from build123d import *

# Parameters (mm, degrees)
EXTRUDE_1_DEPTH     = 1.2
SKETCH_2_R          = 1.375
CUT_EXTRUDE_1_DEPTH = 1.2
SKETCH_3_W          = 6
SKETCH_3_H          = 13
EXTRUDE_2_DEPTH     = 5
SKETCH_4_W          = 6
SKETCH_4_H          = 5
EXTRUDE_3_DEPTH     = 0.3
SKETCH_5_W          = 14.5
SKETCH_5_H          = 7
EXTRUDE_4_DEPTH     = 9
SKETCH_6_W          = 13
SKETCH_6_H          = 6
EXTRUDE_5_DEPTH     = 6
SKETCH_11_W         = 51.4
SKETCH_11_H         = 5.1
EXTRUDE_9_DEPTH     = 8.5
SKETCH_12_W         = 6.2
SKETCH_12_H         = 6.2
EXTRUDE_10_DEPTH    = 3.5
SKETCH_13_R         = 1.75
EXTRUDE_11_DEPTH    = 1.5
SKETCH_15_R         = 2.75
SKETCH_15_R_2       = 1.55
EXTRUDE_13_DEPTH    = 2
SKETCH_16_W         = 51.4
SKETCH_16_H         = 5.1
EXTRUDE_14_DEPTH    = 9


with BuildPart() as part:
    # 草图1 → 凸台-拉伸1 (new body)
    with BuildSketch(Plane(origin=(0, 0, 0), x_dir=(1, 0, 0), z_dir=(0, 1, 0))):
        with BuildLine():
            Line((-29.5, 15), (29.5, 15))
            ThreePointArc((29.5, 15), (31.621320344, 14.121320344), (32.5, 12))
            Line((32.5, 12), (32.5, -12))
            ThreePointArc((32.5, -12), (31.621320344, -14.121320344), (29.5, -15))
            Line((29.5, -15), (-29.5, -15))
            ThreePointArc((-29.5, -15), (-31.621320344, -14.121320344), (-32.5, -12))
            Line((-32.5, -12), (-32.5, 12))
            ThreePointArc((-32.5, 12), (-31.621320344, 14.121320344), (-29.5, 15))
        make_face()
    extrude(amount=EXTRUDE_1_DEPTH)

    # 草图2 → 切除-拉伸1 (cut)
    with BuildSketch(Plane(origin=(0, 1.2, 0), x_dir=(1, 0, 0), z_dir=(0, 1, 0))):
        with Locations(Location((29, -11.5, 0), (0, 0, 270))):
            Circle(SKETCH_2_R)
        with Locations(Location((29, 11.5, 0), (0, 0, 270))):
            Circle(SKETCH_2_R)
        with Locations(Location((-29, -11.5, 0), (0, 0, 270))):
            Circle(SKETCH_2_R)
        with Locations(Location((-29, 11.5, 0), (0, 0, 270))):
            Circle(SKETCH_2_R)
    extrude(amount=-CUT_EXTRUDE_1_DEPTH, mode=Mode.SUBTRACT)

    # 草图3 → 凸台-拉伸2 (add)
    with BuildSketch(Plane(origin=(0, 1.2, 0), x_dir=(1, 0, 0), z_dir=(0, 1, 0))):
        with Locations((21.5, -8.5)):
            Rectangle(SKETCH_3_W, SKETCH_3_H)
    extrude(amount=EXTRUDE_2_DEPTH)

    # 草图4 → 凸台-拉伸3 (add)
    with BuildSketch(Plane.XY.offset(15)):
        with Locations((21.5, 3.7)):
            Rectangle(SKETCH_4_W, SKETCH_4_H)
    extrude(amount=EXTRUDE_3_DEPTH)

    # 草图5 → 凸台-拉伸4 (add)
    with BuildSketch(Plane(origin=(0, 1.2, 0), x_dir=(1, 0, 0), z_dir=(0, 1, 0))):
        with Locations((-0.75, -11.5)):
            Rectangle(SKETCH_5_W, SKETCH_5_H)
    extrude(amount=EXTRUDE_4_DEPTH)

    # 草图6 → 凸台-拉伸5 (add)
    with BuildSketch(Plane(origin=(0, 1.2, 0), x_dir=(1, 0, 0), z_dir=(0, 1, 0))):
        with Locations((-17, -12)):
            Rectangle(SKETCH_6_W, SKETCH_6_H)
    extrude(amount=EXTRUDE_5_DEPTH)

    # 草图11 → 凸台-拉伸9 (add)
    with BuildSketch(Plane.XZ):
        with Locations((-0.05, -11.55)):
            Rectangle(SKETCH_11_W, SKETCH_11_H)
    extrude(amount=EXTRUDE_9_DEPTH)

    # 草图12 → 凸台-拉伸10 (add)
    with BuildSketch(Plane(origin=(0, 1.2, 0), x_dir=(1, 0, 0), z_dir=(0, 1, 0))):
        with Locations((-15.4, 1.4)):
            Rectangle(SKETCH_12_W, SKETCH_12_H)
    extrude(amount=EXTRUDE_10_DEPTH)

    # 草图13 → 凸台-拉伸11 (add)
    with BuildSketch(Plane(origin=(0, 4.7, 0), x_dir=(1, 0, 0), z_dir=(0, 1, 0))):
        with Locations(Location((-15.4, 1.4, 0), (0, 0, 270))):
            Circle(SKETCH_13_R)
    extrude(amount=EXTRUDE_11_DEPTH)

    # 草图15 → 凸台-拉伸13 (add)
    with BuildSketch(Plane.XY.offset(15.3)):
        with Locations(Location((21.5, 3.7, 0), (0, 0, 114.619977329))):
            Circle(SKETCH_15_R)
        with Locations((21.5, 3.7)):
            Circle(SKETCH_15_R_2, mode=Mode.SUBTRACT)
    extrude(amount=EXTRUDE_13_DEPTH)

    # 草图16 → 凸台-拉伸14 (add)
    with BuildSketch(Plane(origin=(0, 1.2, 0), x_dir=(1, 0, 0), z_dir=(0, 1, 0))):
        with Locations((-0.05, 11.55)):
            Rectangle(SKETCH_16_W, SKETCH_16_H)
    extrude(amount=EXTRUDE_14_DEPTH)


solid = part.part
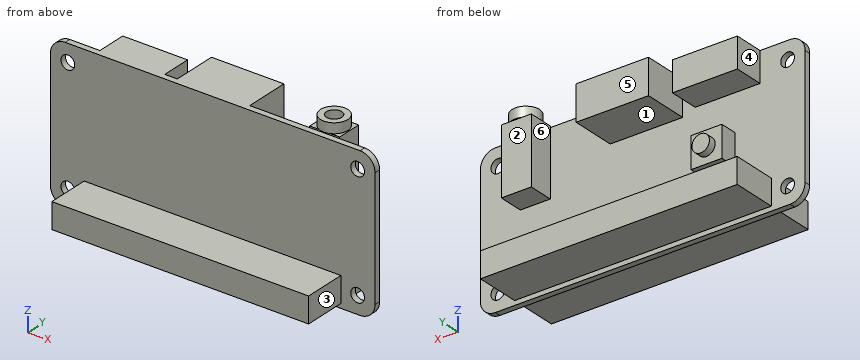
Verification items for the finished model (mm, model axes). Face numbers are marked on the shaded views. A direction names the side the tool comes from. Round coordinates to 2 decimals unless told otherwise and drop trailing zeros. Loops run counter-clockwise (first coordinate to the right, second up) from the corner with the lowest first, then second, coordinate; pieces in that order, holes last. Notation, with made-up numbers: M 27,-9 L 69,-9 A14 cw 69,2 Z; hole C -18.5,11.5 d10. An arc over 180 degrees is marked long. Write each question's results on one line, items separated by ' | '.
1) Section check D-D on y = -6.5. Record the boundary of the cut face in (x, z), then the cut area to 3 significant figures.
Checks:
outline: M -25.75,-14.1 L 25.65,-14.1 L 25.65,-9 L -25.75,-9 Z | area: 262 mm2
2) Section check B-B on z = 5. Record the boundary of the cut face in (x, y).
Checks:
outline: M -32.5,0 L 32.5,0 L 32.5,1.2 L 24.5,1.2 L 24.5,6.2 L 18.5,6.2 L 18.5,1.2 L -32.5,1.2 Z
3) Section check C-C on x = 12.5. Record the boundary of the cut face in (y, z).
Checks:
outline: M -8.5,-14.1 L 0,-14.1 L 0,-15 L 1.2,-15 L 1.2,-14.1 L 10.2,-14.1 L 10.2,-9 L 1.2,-9 L 1.2,15 L 0,15 L 0,-9 L -8.5,-9 Z
4) Mould release check, pull along X, two halves, no side actions. Record for the marked faces 4, 5 and 6: released by +X, released by -X, zero draft, split by the parting line, or undercut.
Checks:
face 4: released by -X | face 5: zero draft | face 6: undercut
5) Access from +Z, -Z, +X, -X, +Y, -Y to the whole of each face (thin tool, end or side, straight path). Record for the marked faces 1, 2 and 3.
Checks:
face 1: -X, +Y | face 2: +X, +Y | face 3: +Z, -Z, +X, -Y
6) Gauge pin test, flat ends, axial feed: P1, Ø4, axis at x = 21.5, y = 3.7, coming from the +Z side; P2, Ø2.5, axis at y = 5.5, z = -11.5, coming from the -X side; P3, Ø3, axis at y = 5.5, z = 12.5, coming from the +X side; P4, Ø2.5, axis at x = 3, y = 5.5, coming from the -Z side. Record the tip position at first contact, or that the pin passes through.
Checks:
P1: stops at z = 17.3 | P2: stops at x = -25.75 | P3: stops at x = 24.5 | P4: stops at z = -14.1
7) Section check A-A on y = 3.7. Record the boundary of the cut face in (x, z).
Checks:
outline: M -25.75,-14.1 L 25.65,-14.1 L 25.65,-9 L -25.75,-9 Z; M -23.5,9 L -10.5,9 L -10.5,15 L -23.5,15 Z; M -18.5,-4.5 L -12.3,-4.5 L -12.3,1.7 L -18.5,1.7 Z; M -8,8 L 6.5,8 L 6.5,15 L -8,15 Z; M 18.5,2 L 24.5,2 L 24.5,15.3 L 24.25,15.3 L 24.25,17.3 L 23.05,17.3 L 23.05,15.3 L 19.95,15.3 L 19.95,17.3 L 18.75,17.3 L 18.75,15.3 L 18.5,15.3 Z
8) Scan lines: L1, parallel to X at y = 5.25, z = 10; L2, parallel to Z at x = -12, y = 3.5; L3, parallel to Y at x = 16, z = -1.5. Record each from-to range of solid material in increasing order. Write a range as from..to.
Checks:
L1: x = -23.5..-10.5, -8..6.5, 18.5..24.5 | L2: z = -14.1..-9, 9..15 | L3: y = 0..1.2
